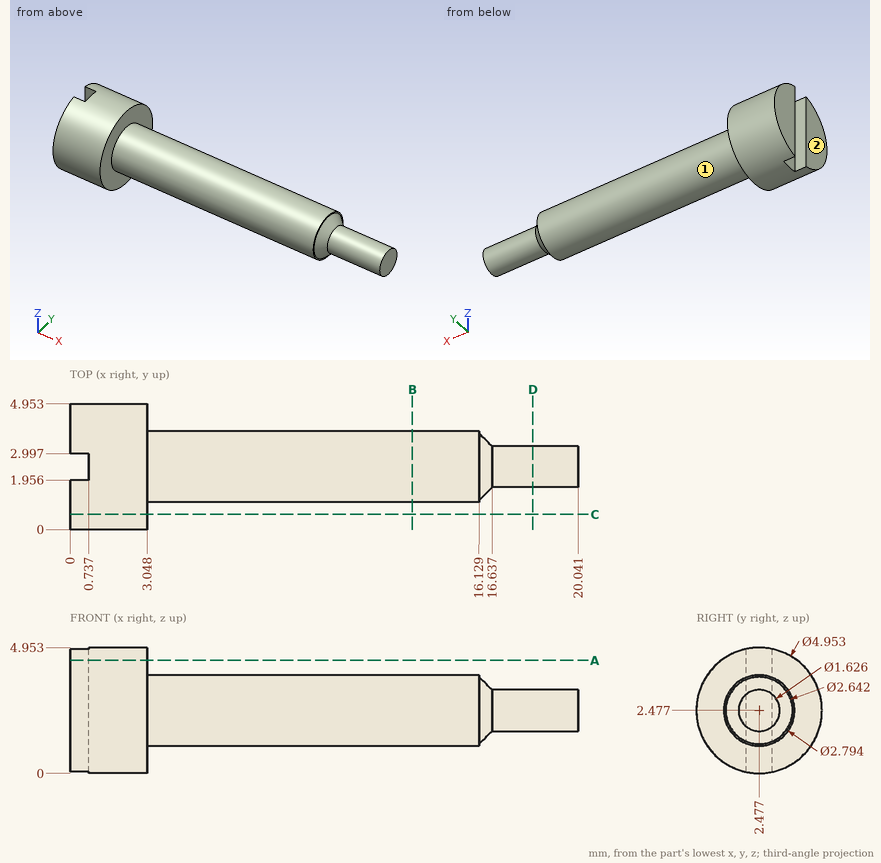
Answer from the drawing. Dimensions are ordinates in mm from the lowest x, y and z of the part. A direction names the side the tool comes from. Give positions to 0.01 mm unless a question says otherwise; leave off trailing zeros. Write each loop counter-clockwise with the first axis right and the second up, starting at its lowest first coordinate (ties: lowest second). Pieces come first, ordered by that corner, then holes. Notation, with made-up numbers: (-26, 89) - (25, 89) arc R12 ccw to (25, 95) - close; hole circle Ø2 at (-9.5, 3.5). An arc over 180 degrees is marked (long way). One line per item, written item: value. Start each with the question number.
1. Consider probe 1 along X at (y, z) = (3.05, 0.95); probe 2 along X at (y, z) = (2.8, 4.05); probe 3 along Z at (x, y) = (13, 2.9) (1 decimal). Determine where each line is inside the solid, lowest interval first.
2. Find section C-C (y = 0.6). Write down the section's boundary in (x, z).
3. For the marked faces 1 and 2, determine the directions among +Z, -Z, +X, -X, +Y, -Y from which every point of the face is accessible in a straight line to the end or side of a thin tool.
4. Find section D-D (x = 18.25). Write down the section's boundary in (y, z) (1 decimal).
5. Given pin 1 (2 mm diameter, centred on x = 7, z = 1, fed in from +Y); pin 2 (0.8 mm diameter, centred on y = 2.5, z = 1.5, fed in from -X); pin 3 (1.5 mm diameter, centred on x = 13, z = 3, fed in from -Y), each flat-ended and moving along its own axis, determine where each tip first touches the part or whether it passes through.
6. Find section A-A (z = 4.45). Write down the section's boundary in (x, y) (1 decimal).
7. Find section B-B (x = 13.5). Write down the section's boundary in (y, z) (1 decimal).
Geometry results:
1. probe 1: 0 to 3.05
1. probe 2: 0.74 to 3.05
1. probe 3: 1.1 to 3.8
2. outline: (0, 0.86) - (3.05, 0.86) - (3.05, 4.09) - (0, 4.09) - close
3. face 1: +X
3. face 2: +Z, -Z, -X, +Y, -Y
4. outline: circle Ø1.6 at (2.5, 2.5)
5. pin 1: y = 3.79
5. pin 2: x = 0.74
5. pin 3: y = 1.08
6. outline: (0, 1) - (3, 1) - (3, 4) - (0, 4) - (0, 3) - (0.7, 3) - (0.7, 2) - (0, 2) - close
7. outline: circle Ø2.8 at (2.5, 2.5)
